Autodesk Inventor part; units mm, degrees
ref_plane "YZ Plane" through (0, 0, 0) normal (1, 0, 0) x (0, 1, 0)
ref_plane "XZ Plane" through (0, 0, 0) normal (0, 1, 0) x (-1, 0, 0)
ref_plane "XY Plane" through (0, 0, 0) normal (0, 0, 1) x (1, 0, 0)
sketch "Sketch1" plane through (0, 0, 0) normal (0, 0, 1) x (1, 0, 0)
  circle A0 centre (0, 0) radius 5
  circle A1 centre (0, 130) radius 5
  circle A2 centre (0, 0) radius 10
  circle A3 centre (0, 130) radius 10
  line L0 (-10, 130) -> (-10, 0)
  line L1 (10, 130) -> (10, 0)
  dimension "d0" = 130
  dimension "d1" = 20
  dimension "d2" = 20
  dimension "d3" = 10
  dimension "d4" = 10
extrude "Extrusion1" add sketch "Sketch1" along normal mid plane 10 contours A0 | A1 | A2 | A2 L0 A3 L1 | A3
sketch "Sketch2" plane through (0, 0, 5) normal (0, 0, 1) x (1, 0, 0)
  arc A0 (10, 130) -> (-10, 130) centre (0, 130) ccw construction
  line L0 (-10, 130) -> (-10, 0) construction
  arc A1 (-10, 0) -> (10, 0) centre (0, 0) ccw construction
  line L1 (10, 0) -> (10, 130) construction
  circle A2 centre (0, 130) radius 5
  circle A3 centre (0, 0) radius 5
  dimension "d7" = 10
  dimension "d8" = 10
extrude "Extrusion2" add sketch "Sketch2" along normal blind 10
fillet "Fillet1" radius 2 2 edges at (-5, 130, 5) (-5, 0, 5)
properties part number "Eslabón 3" material "Steel"
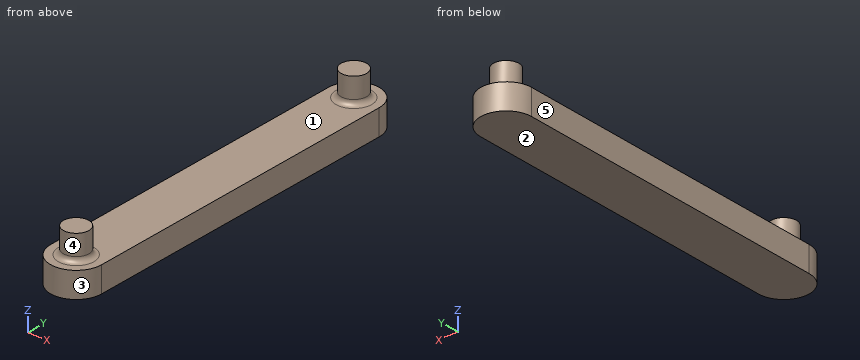
CAD build for the part. Positions are in the model's coordinates, mm. Face numbers are marked on the shaded views. A direction names the side the tool comes from. Give positions to 0.01 mm unless a question says otherwise; leave off trailing zeros. Order: outer loops, then holes, each group sorted by start corner. A loop starts at its lowest first (then second) coordinate and runs counter-clockwise, first axis right, second up. Notation, with made-up numbers: (-37, 20.5) -> (-30, 20.5) arc R36 ccw to (-30, 57.5) -> close; hole circle Ø11 at (27.25, 4). An arc over 180 degrees is marked (long way). Return JSON: item names as keys, results as strings.
Q1. Saw through at C-C (y = 40.5). Write the cut outline in (x, z).
Working result:
{"outline": "(-10, -5) -> (10, -5) -> (10, 5) -> (-10, 5) -> close"}
Q2. Which spindle directions (+Z, -Z, +X, -X, +Y, -Y) get a long thin tool onto all of the face, cutting with end or side? Do the marked faces 4 and 5. Say none if no direction does.
Working result:
{"face 4": "+Z", "face 5": "+Z, -Z, -X, +Y, -Y"}
Q3. Saw through at B-B (z = -2). Write the cut outline in (x, y).
Working result:
{"outline": "(-10, 0) arc R10 ccw to (10, 0) -> (10, 130) arc R10 ccw to (-10, 130) -> close"}
Q4. Flat gauge pins, fed straight in: pin 1 (5 mm diameter, centred on x = 2.5, y = 82.5, fed in from +Z); pin 2 (8 mm diameter, centred on x = -4.5, z = 2, fed in from +Y); pin 3 (1 mm diameter, centred on x = -7.5, z = 2, fed in from -Y). Where does each tip first touch, or does it go through?
Working result:
{"pin 1": "z = 5", "pin 2": "y = 139.99", "pin 3": "y = -7.14"}
Q5. Drill centre lines: line 1 (Z direction, x = -6, y = 59.5); line 2 (Y direction, x = -0.5, z = 6.25); line 3 (Y direction, x = -3, z = 8). Where is each one in solid material? Low to high.
Working result:
{"line 1": "-5 to 5", "line 2": "-5.12 to 5.12, 124.88 to 135.12", "line 3": "-4 to 4, 126 to 134"}
Q6. Saw through at A-A (x = 0). Write the cut outline in (y, z).
Working result:
{"outline": "(-10, -5) -> (140, -5) -> (140, 5) -> (137, 5) arc R2 cw to (135, 7) -> (135, 15) -> (125, 15) -> (125, 7) arc R2 cw to (123, 5) -> (7, 5) arc R2 cw to (5, 7) -> (5, 15) -> (-5, 15) -> (-5, 7) arc R2 cw to (-7, 5) -> (-10, 5) -> close"}
Q7. Mould opens along Y. For the marked faces 1, 2 and 3 say: pulls with the +Y half, pulls with the -Y half, needs draft (parallel to the pull), parting line crosses it, or undercut.
Working result:
{"face 1": "undercut", "face 2": "needs draft", "face 3": "pulls with the -Y half"}
